Autodesk Inventor part; units mm, degrees
ref_plane "YZ Plane" through (0, 0, 0) normal (1, 0, 0) x (0, 1, 0)
ref_plane "XZ Plane" through (0, 0, 0) normal (0, 1, 0) x (-1, 0, 0)
ref_plane "XY Plane" through (0, 0, 0) normal (0, 0, 1) x (1, 0, 0)
sketch "Эскиз1" plane through (0, 0, 0) normal (0, 1, 0) x (-1, 0, 0)
  line L0 (13, -24) -> (-13, -24)
  line L1 (-13, -24) -> (-13, 24)
  line L2 (-13, 24) -> (13, 24)
  line L3 (13, 24) -> (13, -24)
  line L4 (13, -24) -> (-13, 24) construction
  line L5 (-13, -24) -> (13, 24) construction
  point P0 (0, 0)
  dimension "d0" = 26
  dimension "d1" = 48
extrude "Выдавливание1" add sketch "Эскиз1" along normal blind 6
sketch "Эскиз3" plane through (-13, 0, 24) normal (0, 0, 1) x (1, 0, 0)
  arc A0 (24, 4) -> (21, 4) centre (22.5, 3.005) ccw construction
  line L0 (26, 0) -> (26, 6)
  line L1 (21, 6) -> (24, 6)
  line L2 (24, 6) -> (24, 4)
  line L3 (24, 4) -> (21, 4) construction
  line L4 (21, 4) -> (21, 6)
  line L5 (21, 6) -> (24, 4) construction
  line L6 (24, 6) -> (21, 4) construction
  arc A1 (21, 4) -> (24, 4) centre (22.5, 3.005) ccw
  point P0 (13, 0)
  point P1 (22.5, 5)
  point P2 (22.5, 5)
  point P3 (22.5, 5)
  point P4 (22.5, 6)
  dimension "d8" = 3.6
  dimension "d10" = 2
  dimension "d11" = 3
  dimension "d12" = 2
extrude "Выдавливание3" cut sketch "Эскиз3" against normal blind 25
pattern_circular "Круговой массив1" count 2 over 360 about axis through (0, -10, 0) along (0, 1, 0) of "Выдавливание3"
sketch "Эскиз2" plane through (0, 6, 0) normal (0, 1, 0) x (1, 0, 0)
  circle A0 centre (-11.0356, 4.379) radius 4
  line L0 (13, 24) -> (-13, 24)
  point P0 (0, 0)
  dimension "d4" = 8
extrude "Выдавливание2" cut sketch "Эскиз2" against normal blind 6
sketch "Эскиз5" plane through (0, 6, 0) normal (0, 1, 0) x (1, 0, 0)
  line L0 (-13, 24) -> (-13, -24)
  arc A0 (-8, 1.7742) -> (-8, 6.9839) centre (-11.0356, 4.379) ccw
  arc A1 (-13, -4.1856) -> (-13.7446, 1.436) centre (-16.743, -1.8213) ccw
  arc A2 (-13, -6.1738) -> (-7.1165, 3.5787) centre (-23.7825, 6.9821) ccw
  point P0 (0, 0)
  point P1 (-5.684, 5.1513)
  point P2 (-13, 0.5431)
properties part number "ЛЦМК.30000.10.00.01 Згт по одснование"
Source: CAD feature listing. Evaluate the final solid. Frame: model axes, mm. A direction names the side the tool comes from. Give positions to 0.01 mm unless a question says otherwise; leave off trailing zeros. Loops run counter-clockwise (first coordinate to the right, second up) from the corner with the lowest first, then second, coordinate; pieces in that order, holes last. Notation, with made-up numbers: (30.5, -6.5) - (44.5, -6.5) arc R28 ccw to (44.5, 24.5) - close; hole circle Ø4 at (-38.75, 43). An arc over 180 degrees is marked (long way). Use CSV: the item, a comma, the result in double quotes. Start each with the question number.
1. Section D-D (x = 9.5). Output: boundary loops of the cut face in (y, z) (3 decimals).
2. Reachability of faces 1 (the flat face through (-11, 5, -16)), 2 (the flat face through (13, 3, 0)), 3 (the flat face through (11, 5, 12)) from +Z, -Z, +X, -X, +Y, -Y: full face, straight path, thin tool, end or side. Return the list, or none.
3. Section C-C (z = -12). Output: boundary loops of the cut face in (x, y) (3 decimals).
4. Pin query (flat end, axial travel): pin 1 (1.8 mm diameter, centred on x = -9.5, y = 3.5, fed in from -Z); pin 2 (4 mm diameter, centred on x = -0.5, z = 1.5, fed in from -Y); pin 3 (2 mm diameter, centred on x = 9.5, y = 3.005, fed in from +Z). Return the tip coordinate at first contact, or that it passes through.
5. Section B-B (x = -9.5). Output: boundary loops of the cut face in (y, z) (1 decimal).
6. Ray query, L1, parallel to X at y = 5.5, z = 6; L2, parallel to X at y = 5, z = -11; L3, parallel to Y at x = -9.5, z = -0.5 (3 decimals). Return the intervals inside material, ascending.
7. Section A-A (y = 4.5). Output: boundary loops of the cut face in (x, z), then the cut area to 3 significant figures.
8. Draft query along Y for faces 4 (the cylindrical face through (-8.622, 1.434, -0.256)), 5 (the cylindrical face through (9.446, 1.206, 11.675)), 6 (the flat face through (-11, 5, 0)), 7 (the flat face through (0, 0, 0)). Return one class per face: +Y half, -Y half, draft (parallel to the pull), parting line (faces both ways), or undercut.
Response:
1,outline,"(0, -24) - (6, -24) - (6, -1) - (1.205, -1) - (1.205, 24) - (0, 24) - close"
2,face 1,"-Z, +Y"
2,face 2,"+Z, -Z, +X, +Y, -Y"
2,face 3,"+Z, +Y"
3,outline,"(-13, 0) - (13, 0) - (13, 6) - (-8, 6) - (-8, 4) arc R1.8 cw (long way) to (-11, 4) - (-11, 6) - (-13, 6) - close"
4,pin 1,"z = 1"
4,pin 2,"y = 0"
4,pin 3,"z = -1"
5,outline,"(0, -24) - (1.2, -24) - (1.2, -8.1) - (0, -8.1) - close; (0, -0.7) - (1.2, -0.7) - (1.2, 1) - (6, 1) - (6, 24) - (0, 24) - close"
6,L1,"-13 to 8, 11 to 13"
6,L2,"-13 to -11, -8 to 13"
6,L3,"0 to 1.205"
7,outline,"(-13, -24) - (-11, -24) - (-11, -8.38) arc R4 cw to (-13, -7.86) - close; (-13, -0.89) arc R4 cw to (-11, -0.38) - (-11, 1) - (-8, 1) - (-8, -1.77) arc R4 cw to (-8, -6.98) - (-8, -24) - (13, -24) - (13, 24) - (11, 24) - (11, -1) - (8, -1) - (8, 24) - (-13, 24) - close"
7,area,"1,080 mm²"
8,face 4,"undercut"
8,face 5,"undercut"
8,face 6,"draft"
8,face 7,"-Y half"
